Geometry check sheet. Reference: the model listing, model coordinates, mm. Face numbers are marked on the shaded views. Give positions to 0.01 mm unless a question says otherwise; leave off trailing zeros. Write each loop counter-clockwise with the first axis right and the second up, starting at its lowest first coordinate (ties: lowest second). Pieces come first, ordered by that corner, then holes. Notation, with made-up numbers: (34.25, 83.25) - (55.25, 83.25) arc R29 ccw to (55.25, 107.25) - close; hole circle Ø7 at (30.5, 59). An arc over 180 degrees is marked (long way). Use a Markdown table: item, result.
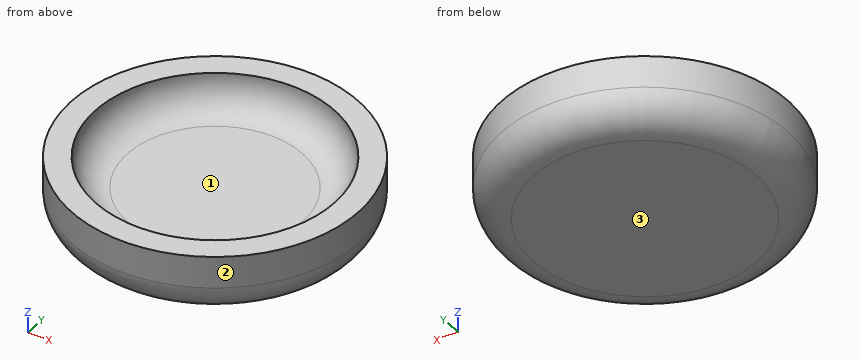
```python
from build123d import *

# Parameters (mm, degrees)
SKETCH1_R           = 9
BOSS_EXTRUDE1_DEPTH = 4
SKETCH2_R           = 7.5
CUT_EXTRUDE1_DEPTH  = 2
FILLET1_R           = 2
FILLET2_R           = 2


with BuildPart() as part:
    # Sketch1 → Boss-Extrude1 (new body)
    with BuildSketch(Plane.XY):
        Circle(SKETCH1_R)
    extrude(amount=BOSS_EXTRUDE1_DEPTH)

    # Sketch2 → Cut-Extrude1 (cut)
    with BuildSketch(Plane.XY.offset(4)):
        Circle(SKETCH2_R)
    extrude(amount=-CUT_EXTRUDE1_DEPTH, mode=Mode.SUBTRACT)

    # Fillet1
    fillet1_edges = [part.edges().sort_by_distance(p)[0] for p in [
        (-9, 0, 0),
    ]]
    fillet(fillet1_edges, radius=FILLET1_R)

    # Fillet2
    fillet2_edges = [part.edges().sort_by_distance(p)[0] for p in [
        (-7.5, 0, 2),
    ]]
    fillet(fillet2_edges, radius=FILLET2_R - 0.0001)  # a hair under: the kernel refuses the full size


solid = part.part
```
1) Material ranges on L1, parallel to Z at x = 2.25, y = -0.5; L2, parallel to X at y = -5, z = 2.6; L3, parallel to Y at x = 4.25, z = 2.9, recorded low to high. Write a range as from..to.
Working result:
| item | result |
|---|---|
| L1 | z = 0..2 |
| L2 | x = -7.48..-4.8, 4.8..7.48 |
| L3 | y = -7.93..-5.78, 5.78..7.93 |
2) Depth check by flat-ended pin: P1, Ø5.5, axis at x = -1, y = 0, coming from the +Z side; P2, Ø2, axis at y = 3.5, z = 3, coming from the -X side. Enter the tip coordinate at first touch or a pass-through.
Working result:
| item | result |
|---|---|
| P1 | stops at z = 2 |
| P2 | stops at x = -8.65 |
3) Section check C-C on z = 3.1. Record the boundary of the cut face in (x, y), then the cut area to 3 significant figures.
Working result:
| item | result |
|---|---|
| outline | circle Ø18 at (0, 0); hole circle Ø14.57 at (0, 0) |
| area | 87.7 mm² |
4) Mould release check, pull along Y, two halves, no side actions. Record for the marked faces 1, 2 and 3: pulls with the +Y half, pulls with the -Y half, needs draft (parallel to the pull), parting line crosses it, or undercut.
Working result:
| item | result |
|---|---|
| face 1 | undercut |
| face 2 | parting line crosses it |
| face 3 | needs draft |
5) Section check D-D on z = 0.85. Record the boundary of the cut face in (x, y).
Working result:
| item | result |
|---|---|
| outline | circle Ø17.27 at (0, 0) |
